Source: CAD feature listing. Evaluate the final solid. Frame: model axes, mm. A direction names the side the tool comes from. Round coordinates to 2 decimals unless told otherwise and drop trailing zeros. Order: outer loops, then holes, each group sorted by start corner. A loop starts at its lowest first (then second) coordinate and runs counter-clockwise, first axis right, second up. Notation, with made-up numbers: (-11.5, 81) -> (15.5, 81) arc R29 cw to (15.5, 102) -> close; hole circle Ø11 at (72, 35.5). An arc over 180 degrees is marked (long way). Answer as CSV lines item,"result". Start each with the question number.
(1) Section query D-D (z = -481.5). Output: boundary loops of the cut face in (x, y).
(2) Line query: line 1 along Y through (x, z) = (161, -470.5); line 2 along X through (y, z) = (27, -519.5); line 3 along Z through (x, y) = (172.25, 26). Output: solid intervals per line, ascending. Write a range as from..to.
(3) Section query C-C (y = 26.5). Count the separate pieces of the cut face and the enclosed holes in it, plus the area to 3 significant figures.
(4) Contact query for flat-ended pins moving along their axis: P1, Ø8, axis at x = 158.5, z = -489.5, coming from the -Y side; P2, Ø4, axis at x = 175.5, y = 28.5, coming from the +Z side; P3, Ø4, axis at y = 28, z = -508.5, coming from the -X side. Output: stop coordinate, or through.
(5) Set-up query: faces 1 (the cylindrical face through (165.844, 26.958, -487.358)), 2 (the flat face through (170, 23, -505)). Return all of +Z, -Z, +X, -X, +Y, -Y with unobstructed straight access to the full face (end or side cutting, diameter ignored); none if empty.
(6) Section query B-B (x = 172.75). Output: boundary loops of the cut face in (y, z).
(7) Section query A-A (z = -497). Output: boundary loops of the cut face in (x, y).
(8) Pull-direction query (Z, two-part tool) for faces 3 (the flat face through (158.32, 26.96, -440.67)), 4 (the flat face through (164.116, 26.958, -463.814)), 5 (the flat face through (161, 24, -460)), 6 (the cylindrical face through (164.05, 27.04, -428.79)); classes: +Z half, -Z half, draft (parallel to the pull), parting line (faces both ways), or undercut.
```python
from build123d import *

# Parameters (mm, degrees)
BOSS_EXTRUDE1_DEPTH = 50
SKETCH2_R           = 10
CUT_EXTRUDE1_DEPTH  = 145
SKETCH3_R           = 10
CUT_EXTRUDE2_DEPTH  = 145
SCALE1_SCALE        = 0.2
BOSS_EXTRUDE2_START = -10
SKETCH4_R           = 2
BOSS_EXTRUDE2_DEPTH = 10
CUT_EXTRUDE3_DEPTH  = 4
SKETCH6_R           = 2
BOSS_EXTRUDE3_DEPTH = 6
BOSS_EXTRUDE4_DEPTH = 1
CUT_EXTRUDE4_DEPTH  = 10
LPATTERN1_COUNT     = 5
LPATTERN1_PITCH     = 5.2


with BuildPart() as part:
    # Sketch1 → Boss-Extrude1 (new body)
    with BuildSketch(Plane(origin=(0, 0, 0), x_dir=(1, 0, 0), z_dir=(0, 1, 0))):
        with BuildLine():
            Line((156.72428326, 188.749431717), (104.362522104, 384.675710784))
            ThreePointArc((104.362522104, 384.675710784), (100.737911875, 412.774532685), (104.619514578, 440.839007595))
            Line((104.619514578, 440.839007595), (155.108674524, 623.056486958))
            ThreePointArc((155.108674524, 623.056486958), (161.096577838, 637.255812747), (170.503706822, 649.461621332))
            Line((170.503706822, 649.461621332), (236.039412862, 714.997327373))
            Line((236.039412862, 714.997327373), (236.039412862, 577.933775776))
            Line((236.039412862, 577.933775776), (180.600392658, 532.253421954))
            ThreePointArc((180.600392658, 532.253421954), (168.395698805, 518.565657016), (160.895546094, 501.83074828))
            Line((160.895546094, 501.83074828), (142.173951469, 433.630653577))
            ThreePointArc((142.173951469, 433.630653577), (140.038780006, 418.542072662), (141.773673112, 403.40224515))
            Line((141.773673112, 403.40224515), (186.844856765, 220.358050312))
            ThreePointArc((186.844856765, 220.358050312), (180.4464863, 196.299603446), (156.72428326, 188.749431717))
        make_face()
    extrude(amount=BOSS_EXTRUDE1_DEPTH)

    # Sketch2 → Cut-Extrude1 (cut)
    with BuildSketch(Plane(origin=(0, 50, 0), x_dir=(1, 0, 0), z_dir=(0, 1, 0))):
        with Locations(Location((120.492692433, 416.694560019, 0), (0, 0, 270))):
            Circle(SKETCH2_R)
    extrude(amount=-CUT_EXTRUDE1_DEPTH, mode=Mode.SUBTRACT)

    # Sketch3 → Cut-Extrude2 (cut)
    with BuildSketch(Plane(origin=(0, 50, 0), x_dir=(1, 0, 0), z_dir=(0, 1, 0))):
        with Locations(Location((165.652720942, 217.997652258, 0), (0, 0, 270))):
            Circle(SKETCH3_R)
    extrude(amount=-CUT_EXTRUDE2_DEPTH, mode=Mode.SUBTRACT)


with BuildPart() as part_1:
    # Scale1: scaled about (165.170943501, 25, -479.501481674)
    add(part.part.scale(SCALE1_SCALE).moved(Location((132.136754801, 20, -383.601185339))))

    # Sketch4 → Boss-Extrude2 (add)
    with BuildSketch(Plane(origin=(0, 30, 0), x_dir=(1, 0, 0), z_dir=(0, 1, 0)).offset(BOSS_EXTRUDE2_START)):
        with BuildLine():
            Line((167.333433502, 464.60578312), (160.807348984, 462.998857787))
            Line((160.807348984, 462.998857787), (160.491489423, 464.281634369))
            ThreePointArc((160.491489423, 464.281634369), (160.144510802, 467.309599871), (160.571545095, 470.327316054))
            Line((160.571545095, 470.327316054), (161.32024353, 473.054717497))
            Line((161.32024353, 473.054717497), (167.42312855, 471.379415727))
            ThreePointArc((167.42312855, 471.379415727), (169.9963123, 467.957931993), (167.333433502, 464.60578312))
        make_face()
        with Locations(Location((166.496619113, 468.004274209, 0), (0, 0, 270))):
            Circle(SKETCH4_R, mode=Mode.SUBTRACT)
    extrude(amount=BOSS_EXTRUDE2_DEPTH)

    # Sketch5 → Cut-Extrude3 (cut)
    with BuildSketch(Plane.XZ.offset(-20)):
        with BuildLine():
            Line((167.333433502, -464.60578312), (160.807348984, -462.998857787))
            Line((160.807348984, -462.998857787), (169.505726154, -427.672795401))
            ThreePointArc((169.505726154, -427.672795401), (168.226052061, -422.861106028), (163.481611453, -421.351071682))
            Line((163.481611453, -421.351071682), (153.009259222, -460.536327496))
            ThreePointArc((153.009259222, -460.536327496), (152.284337176, -466.156091876), (153.060657717, -471.768986858))
            Line((153.060657717, -471.768986858), (163.158489706, -508.21248273))
            ThreePointArc((163.158489706, -508.21248273), (164.356070369, -511.052347888), (166.237496165, -513.493509605))
            Line((166.237496165, -513.493509605), (179.344637373, -526.600650813))
            Line((179.344637373, -526.600650813), (179.344637373, -499.187940494))
            Line((179.344637373, -499.187940494), (168.256833333, -490.05186973))
            ThreePointArc((168.256833333, -490.05186973), (165.815894562, -487.314316742), (164.31586402, -483.967334995))
            Line((164.31586402, -483.967334995), (161.32024353, -473.054717497))
            Line((161.32024353, -473.054717497), (167.42312855, -471.379415727))
            ThreePointArc((167.42312855, -471.379415727), (169.9963123, -467.957931993), (167.333433502, -464.60578312))
        make_face()
    extrude(amount=-CUT_EXTRUDE3_DEPTH, mode=Mode.SUBTRACT)

    # Sketch6 → Boss-Extrude3 (add)
    with BuildSketch(Plane(origin=(0, 30, 0), x_dir=(1, 0, 0), z_dir=(0, 1, 0))):
        with Locations((156.235293288, 466.940097343)):
            Circle(SKETCH6_R)
    extrude(amount=-BOSS_EXTRUDE3_DEPTH)

    # Sketch7 → Boss-Extrude4 (add)
    with BuildSketch(Plane(origin=(0, 30, 0), x_dir=(1, 0, 0), z_dir=(0, 1, 0))):
        with BuildLine():
            Line((179.344637373, 526.600650813), (166.237496165, 513.493509605))
            ThreePointArc((166.237496165, 513.493509605), (164.356070369, 511.052347888), (163.158489706, 508.21248273))
            Line((163.158489706, 508.21248273), (160.776954555, 499.617423264))
            ThreePointArc((160.776954555, 499.617423264), (162.10559666, 492.949108842), (168.256833333, 490.05186973))
            Line((168.256833333, 490.05186973), (179.344637373, 499.187940494))
            Line((179.344637373, 499.187940494), (179.344637373, 526.600650813))
        make_face()
    boss_extrude4 = extrude(amount=BOSS_EXTRUDE4_DEPTH)

    # Mirror2: Boss-Extrude4 across plane
    add(boss_extrude4.mirror(Plane.ZX.offset(27)))

    # Sketch8 → Cut-Extrude4 (cut)
    with BuildSketch(Plane(origin=(0, 31, 0), x_dir=(1, 0, 0), z_dir=(0, 1, 0))):
        Polygon((178.344637373, 500.614741506), (179.344637373, 499.187940494), (179.344637373, 501.787940494), align=None)
        Polygon((178.344637373, 503.214741506), (179.344637373, 501.787940494), (179.344637373, 504.387940494), align=None)
    cut_extrude4 = extrude(amount=-CUT_EXTRUDE4_DEPTH, mode=Mode.SUBTRACT)

    # LPattern1: Cut-Extrude4 ×5
    with Locations(*[(0, 0, -i * LPATTERN1_PITCH) for i in range(1, LPATTERN1_COUNT)]):
        add(cut_extrude4, mode=Mode.SUBTRACT)


solid = part_1.part
```
Answer block:
1,outline,"(155.76, 24) -> (163.64, 24) -> (163.64, 30) -> (155.76, 30) -> close"
2,line 1,"24..30"
2,line 2,"172.24..178.93"
2,line 3,"-519.51..-493.34"
3,separate pieces,"1"
3,enclosed holes,"2"
3,area,"1,030 mm2"
4,P1,"y = 24"
4,P2,"z = -494.37"
4,P3,"x = 162.68"
5,face 1,"+X, +Y, -Y"
5,face 2,"+Z, -Z, +X, -X, -Y"
6,outline,"(23, -520.01) -> (31, -520.01) -> (31, -493.75) -> (23, -493.75) -> close"
7,outline,"(160.05, 24) -> (160.53, 24) -> (160.53, 23) -> (176.69, 23) -> (176.69, 31) -> (160.53, 31) -> (160.53, 30) -> (160.05, 30) -> close"
8,face 3,"+Z half"
8,face 4,"undercut"
8,face 5,"draft"
8,face 6,"undercut"
